```python
from build123d import *

# Parameters (mm, degrees)
F2_S5_R     = 3.048
F2_T6_DEPTH = 6


# Not quite as in the source:
# - a fillet or chamfer that OpenCascade refuses, or shapes differently, is made with other operations: its cross-section is extruded or revolved along the edge and cut away or added


with BuildPart() as f1:
    # F0 (on Right) → F1 (revolve)
    with BuildSketch(Plane.YZ):
        Polygon((0, 57.15), (0, 0), (4.7625, 0), (4.7625, 4.6736), (3.175, 4.6736), (3.175, 37.9984), (3.048, 37.9984), (3.048, 57.15), align=None)
    revolve(axis=Axis((0, 0, 28.575), (0, 0, -1)))

    # F2: chamfer of 0.254 on 1 edges, made by hand


with BuildPart() as f2_tool2:
    # F2_s3 → F2_t4 (revolve)
    with BuildSketch(Plane.YZ):
        Polygon((3.175, 37.7444), (2.921, 37.9984), (3.175, 37.9984), align=None)
    revolve(axis=Axis((0, 0, 37.9984), (0, 0, -1)))

    # F2_s5 → F2_t6 (cut, symmetric)
    with BuildSketch(Plane.XY.offset(37.9)):
        Circle(F2_S5_R)
    extrude(amount=F2_T6_DEPTH, both=True, mode=Mode.SUBTRACT)


with BuildPart() as f1_1:
    add(f1.part)

    # F2_t1: cut F2_tool2
    add(f2_tool2.part, mode=Mode.SUBTRACT)


solid = f1_1.part
```
Input: part model. Units: mm. Frame: model coordinates. A direction names the side the tool comes from. Coordinates: 2 decimals unless noted, no trailing zeros. Write each loop counter-clockwise with the first axis right and the second up, starting at its lowest first coordinate (ties: lowest second). Pieces come first, ordered by that corner, then holes.
1) Set-up query: faces 1 (the flat face through (0, 0, 57.15)), 2 (the cylindrical face through (-3.1, -0.69, 21.44)). Return all of +Z, -Z, +X, -X, +Y, -Y with unobstructed straight access to the full face (end or side cutting, diameter ignored); none if empty.
2) Material intervals for line 1 along X through (y, z) = (-0.25, 42); line 2 along Z through (x, y) = (3, 3.5); line 3 along X through (y, z) = (0.25, 36.5), sorted ascending.
3) Pin query (flat end, axial travel): pin 1 Ø1.5 at (x, z) = (-2, 26) entering from -Y; pin 2 Ø1 at (x, z) = (-3, 7) entering from -Y; pin 3 Ø1.5 at (x, z) = (-1, 10.5) entering from -Y. Return the tip coordinate at first contact, or that it passes through.
4) Section C-C on z = 31. Output: boundary loops of the cut face in (x, y) (3 decimals).
Check result:
1. face 1: +Z, +X, -X, +Y, -Y
1. face 2: +Z
2. line 1: x = -3.04 to 3.04
2. line 2: z = 0 to 4.67
2. line 3: x = -3.17 to 3.17
3. pin 1: stops at y = -2.92
3. pin 2: stops at y = -1.96
3. pin 3: stops at y = -3.17
4. outline: circle Ø6.35 at (0, 0)
